The listing builds one solid part. Answer for the finished solid, in the listing's coordinates (mm). Face numbers are marked on the shaded views. Coordinates: 2 decimals unless noted, no trailing zeros. Order: outer loops, then holes, each group sorted by start corner. A loop starts at its lowest first (then second) coordinate and runs counter-clockwise, first axis right, second up. Notation, with made-up numbers: (18, 9.25) -> (73, 9.25) arc R10 cw to (73, 17.25) -> close; hole circle Ø9 at (35.25, 16.5). An arc over 180 degrees is marked (long way). Return JSON: item names as keys, results as strings.
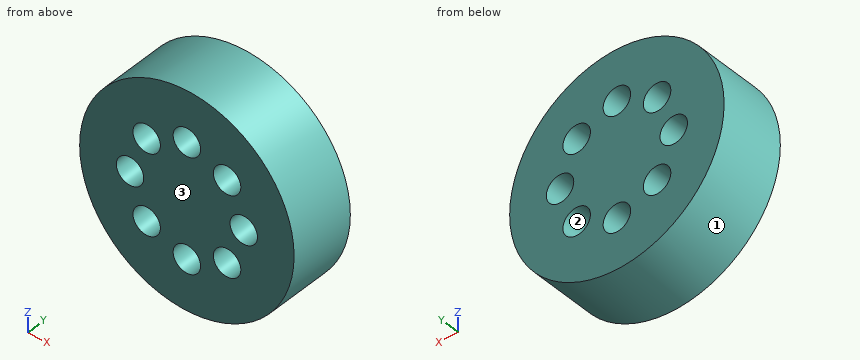
Autodesk Inventor part; units mm, degrees
ref_plane "YZ Plane" through (0, 0, 0) normal (1, 0, 0) x (0, 1, 0)
ref_plane "XZ Plane" through (0, 0, 0) normal (0, 1, 0) x (-1, 0, 0)
ref_plane "XY Plane" through (0, 0, 0) normal (0, 0, 1) x (1, 0, 0)
sketch "Sketch1" plane through (0, 0, 0) normal (0, 1, 0) x (-1, 0, 0)
  circle A0 centre (0, 0) radius 16
  circle A1 centre (0, 0) radius 2.5 construction
  circle A2 centre (6, 6) radius 2.05
  circle A3 centre (0, 8.4853) radius 2.05
  circle A4 centre (-6, 6) radius 2.05
  circle A5 centre (-8.4853, 0) radius 2.05
  circle A6 centre (-6, -6) radius 2.05
  circle A7 centre (0, -8.4853) radius 2.05
  circle A8 centre (6, -6) radius 2.05
  circle A9 centre (8.4853, 0) radius 2.05
  dimension "d0" = 32
  dimension "d1" = 5
  dimension "d2" = 4.1
  dimension "d3" = 6
  dimension "d4" = 6
  dimension "d7" = 360
extrude "Extrusion1" add sketch "Sketch1" along normal mid plane 10
properties part number "PulleySpacer"
Item 1: The part is cut by section A-A on z = 0. Determine the outline of the cut face in (x, y), plus the area to 3 significant figures.
Answer list:
{"outline": "(-16, -5) -> (-10.54, -5) -> (-10.54, 5) -> (-16, 5) -> close; (-6.44, -5) -> (6.44, -5) -> (6.44, 5) -> (-6.44, 5) -> close; (10.54, -5) -> (16, -5) -> (16, 5) -> (10.54, 5) -> close", "area": "238 mm2"}
Item 2: Find the intervals of material crossed by probe 1 along Z at (x, y) = (0, 2); probe 2 along Z at (x, y) = (6, -3.5); probe 3 along X at (y, z) = (4.25, 1.5), in increasing order.
Answer list:
{"probe 1": "-16 to -10.54, -6.44 to 6.44, 10.54 to 16", "probe 2": "-14.83 to -8.05, -3.95 to 3.95, 8.05 to 14.83", "probe 3": "-15.93 to -9.88, -7.09 to 7.09, 9.88 to 15.93"}
Item 3: Determine the mould class of the marked faces 1, 2 and 3 for opening direction X: pulls with the +X half, pulls with the -X half, needs draft (parallel to the pull), parting line crosses it, or undercut.
Answer list:
{"face 1": "parting line crosses it", "face 2": "undercut", "face 3": "needs draft"}
Item 4: The part is cut by section C-C on y = 1.75. Count the separate pieces of the cut face and the enclosed holes in it, plus the area to 3 significant figures.
Answer list:
{"separate pieces": "1", "enclosed holes": "8", "area": "699 mm2"}
Item 5: Flat-ended cylindrical pins translate along their axes: pin 1 (4.5 mm diameter, centred on x = 6, z = 6, fed in from +Y); pin 2 (5 mm diameter, centred on x = -3.5, y = -3.5, fed in from +Z); pin 3 (1 mm diameter, centred on y = 1, z = 3.5, fed in from -X); pin 4 (1.5 mm diameter, centred on y = 3.5, z = -8.5, fed in from -X). Find the tip coordinate at first contact, or state that the pin passes through.
Answer list:
{"pin 1": "y = 5", "pin 2": "z = 15.97", "pin 3": "x = -15.72", "pin 4": "x = -14"}
Item 6: The part is cut by section D-D on x = -9. Determine the outline of the cut face in (y, z).
Answer list:
{"outline": "(-5, -13.23) -> (5, -13.23) -> (5, -1.98) -> (-5, -1.98) -> close; (-5, 1.98) -> (5, 1.98) -> (5, 13.23) -> (-5, 13.23) -> close"}
Item 7: The part is cut by section B-B on x = 0. Determine the outline of the cut face in (y, z), plus the area to 3 significant figures.
Answer list:
{"outline": "(-5, -16) -> (5, -16) -> (5, -10.54) -> (-5, -10.54) -> close; (-5, -6.44) -> (5, -6.44) -> (5, 6.44) -> (-5, 6.44) -> close; (-5, 10.54) -> (5, 10.54) -> (5, 16) -> (-5, 16) -> close", "area": "238 mm2"}
